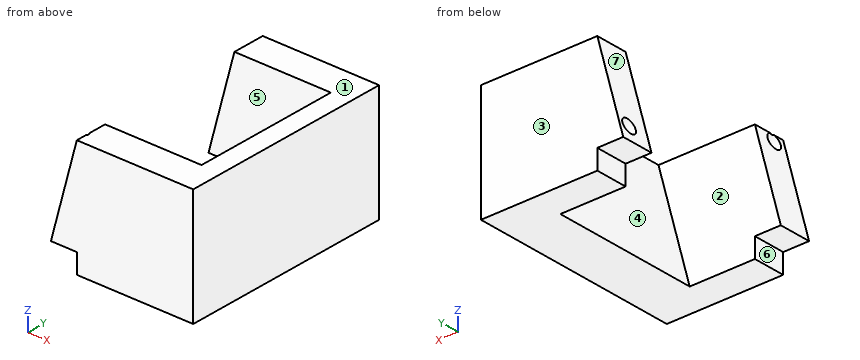
```python
from build123d import *

# Parameters (mm, degrees)
F1_DEPTH = 46
F3_W     = 46
F3_H     = 25
F5_DEPTH = 25
F4_W     = 32
F4_H     = 45
F6_DEPTH = 20
F2_R     = 1.65
F7_DEPTH = 20


with BuildPart() as f1:
    # F0 (on Front) → F1 (new body)
    with BuildSketch(Plane.XZ):
        Polygon((-5.564609, 0), (0, 0), (0, 20.767405), align=None)
    extrude(amount=F1_DEPTH)

    # F3 (on face) → F5 (join)
    with BuildSketch(Plane.YZ):
        with Locations((-23, 8.267405)):
            Rectangle(F3_W, F3_H)
    extrude(amount=F5_DEPTH)

    # F4 (on face) → F6 (cut)
    with BuildSketch(Plane(origin=(-5.191851, 0, 1.391152), x_dir=(0, -1, 0), z_dir=(-0.965926, 0, 0.258819))):
        with Locations((23, 10.834288)):
            Rectangle(F4_W, F4_H)
    extrude(amount=-F6_DEPTH, mode=Mode.SUBTRACT)

    # F2 (on face) → F7 (cut)
    with BuildSketch(Plane(origin=(-5.191851, 0, 1.391152), x_dir=(0, -1, 0), z_dir=(-0.965926, 0, 0.258819))):
        with Locations((2.5, 2.059773)):
            Circle(F2_R)
        with Locations((43.3, 18.459773)):
            Circle(F2_R)
    extrude(amount=-F7_DEPTH, mode=Mode.SUBTRACT)


solid = f1.part
```
Work out the finished part from the listing and answer in its coordinate system (mm). Face numbers are marked on the shaded views. A direction names the side the tool comes from. Round coordinates to 2 decimals unless told otherwise and drop trailing zeros. Order: outer loops, then holes, each group sorted by start corner. A loop starts at its lowest first (then second) coordinate and runs counter-clockwise, first axis right, second up.
Q1. The mould has two halves that part along Y. Classify the marked faces 1, 2, 3 and 4: pulls with the +Y half, pulls with the -Y half, needs draft (parallel to the pull), parting line crosses it, or undercut.
Solution:
face 1: needs draft
face 2: undercut
face 3: pulls with the +Y half
face 4: undercut
Q2. A tool of negligible diameter and unlimited length cuts with its end or side. For the marked faces 5, 6 and 7, from which of +Z, -Z, +X, -X, +Y, -Y can it reach the whole face along a straight path? Write none if from no direction.
Solution:
face 5: +Z, -X
face 6: -Z, -X, +Y, -Y
face 7: +Z, -X, +Y, -Y
Q3. A cutting plane is placed at C-C, the plane y = -6. Determine the outline of the cut face in (x, z), then the cut area to 3 significant figures.
Solution:
outline: (-5.56, 0) - (0, 0) - (0, -4.23) - (25, -4.23) - (25, 20.77) - (0, 20.77) - close
area: 683 mm2
Q4. A cutting plane is placed at B-B, the plane x = 7.5. Count the separate pieces of the cut face and the enclosed holes in it, then the cut area to 3 significant figures.
Solution:
separate pieces: 2
enclosed holes: 2
area: 332 mm2
Q5. A cutting plane is placed at A-A, the plane z = 6.25. Determine the outline of the cut face in (x, y).
Solution:
outline: (-3.89, -46) - (25, -46) - (25, 0) - (-3.89, 0) - (-3.89, -7) - (16.82, -7) - (16.82, -39) - (-3.89, -39) - close
Q6. Given pin 1 Ø3 at (x, y) = (-2.5, -4.5) entering from -Z; pin 2 Ø3.5 at (y, z) = (-43.5, -2) entering from -X, each flat-ended and moving along its own axis, determine where each tip first touches the part or whether it passes through.
Solution:
pin 1: stops at z = 0
pin 2: stops at x = 0
Q7. Find the intervals of material crossed by line 1 along Y through (x, z) = (17.5, 16.25); line 2 along Y through (x, z) = (2, 17.25); line 3 along Y through (x, z) = (2.5, 2), in increasing order.
Solution:
line 1: y = -46 to -39, -7 to 0
line 2: y = -46 to -44.34, -42.26 to -39, -7 to 0
line 3: y = -46 to -39, -7 to -4.07, -0.93 to 0
